Here's how the part is built. I have some questions about the finished solid (model axes, mm). Face numbers are marked on the shaded views. A direction names the side the tool comes from. Give positions to 0.01 mm unless a question says otherwise; leave off trailing zeros. Write each loop counter-clockwise with the first axis right and the second up, starting at its lowest first coordinate (ties: lowest second). Pieces come first, ordered by that corner, then holes. Notation, with made-up numbers: (-37.75, 11.25) - (7.25, 11.25) arc R25 ccw to (7.25, 40.25) - close; hole circle Ø9 at (-15.75, 13). An arc over 180 degrees is marked (long way). One line per item, written item: value. Start each with the question number.
1) Please list where these lines run through material, in increasing order: L1, parallel to Z at x = 3, y = 0; L2, parallel to X at y = 1.5, z = 3; L3, parallel to Y at x = 2, z = 1. Write a range as [from, to].
2) Imagine slicing it at A-A on x = 3. Write out the boundary of the cut face in (y, z), plus the area to 3 significant figures.
3) I'm going to push flat-ended pins straight in: P1, Ø2, axis at x = 29.5, y = -1.5, coming from the -Z side; P2, Ø3, axis at x = 18.5, z = -2.5, coming from the -Y side; P3, Ø5, axis at x = 17.5, y = -3.5, coming from the +Z side. Where does each tip first touch, or does it pass through?
4) Imagine slicing it at B-B on x = 28. Write out the boundary of the cut face in (y, z).
5) On a 3-axis mill with a long thin cutter (end or side, diameter ignored), from which of +Z, -Z, +X, -X, +Y, -Y can I reach the whole of each face in a straight line? I mean the marked faces 1 and 2. Say none if no direction works.
6) We'd pull the mould along Z, two halves only. Please class the marked faces 3, 4 and 5: +Z half, -Z half, draft (parallel to the pull), parting line (faces both ways), or undercut.
7) Imagine slicing it at C-C on z = 3. Write out the boundary of the cut face in (x, y).
from build123d import *

# Parameters (mm, degrees)
M5_GEWINDEBOHRUNG1_D     = 4.2
M5_GEWINDEBOHRUNG1_DEPTH = 14
M5_GEWINDEBOHRUNG1_TIP   = 1.2618073


with BuildPart() as part:
    # Skizze1 → Rotation1 (revolve)
    with BuildSketch(Plane.XY):
        Polygon((0, 0), (0, 5), (36, 5), (36, 2.5), (44, 2.5), (44, 0), align=None)
    revolve(axis=Axis((0, 0, 0), (1, 0, 0)))

    # M5 Gewindebohrung1
    with Locations(Plane.ZY):
        with Locations((0, 0)):
            Hole(M5_GEWINDEBOHRUNG1_D / 2, depth=M5_GEWINDEBOHRUNG1_DEPTH)
            with Locations((0, 0, -(M5_GEWINDEBOHRUNG1_DEPTH + M5_GEWINDEBOHRUNG1_TIP / 2))):  # 118° drill point
                Cone(0, M5_GEWINDEBOHRUNG1_D / 2, M5_GEWINDEBOHRUNG1_TIP, mode=Mode.SUBTRACT)


solid = part.part
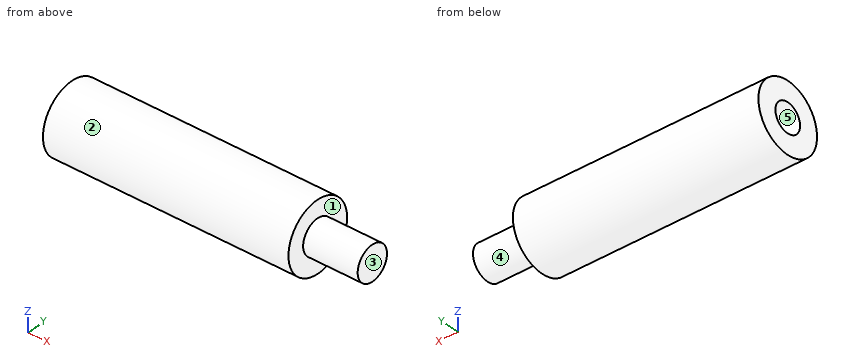
Numbers:
1. L1: [-5, -2.1], [2.1, 5]
1. L2: [0, 36]
1. L3: [-4.9, -1.85], [1.85, 4.9]
2. outline: circle Ø10 at (0, 0); hole circle Ø4.2 at (0, 0)
2. area: 64.7 mm^2
3. P1: z = -4.97
3. P2: y = -4.9
3. P3: z = 4.9
4. outline: circle Ø10 at (0, 0)
5. face 1: +X
5. face 2: +X, -X
6. face 3: draft
6. face 4: parting line
6. face 5: undercut
7. outline: (0, -4) - (36, -4) - (36, 4) - (0, 4) - close
